Verification items for this drawing (mm, ordinates from the low corner). A direction names the side the tool comes from. Round coordinates to 2 decimals unless told otherwise and drop trailing zeros. Loops run counter-clockwise (first coordinate to the right, second up) from the corner with the lowest first, then second, coordinate; pieces in that order, holes last. Notation, with made-up numbers: (-20.75, 56.25) - (8.25, 56.25) arc R17 cw to (8.25, 80.25) - close; hole circle Ø7 at (14.5, 34.5). An arc over 180 degrees is marked (long way). Put each result on its own line as item: value.
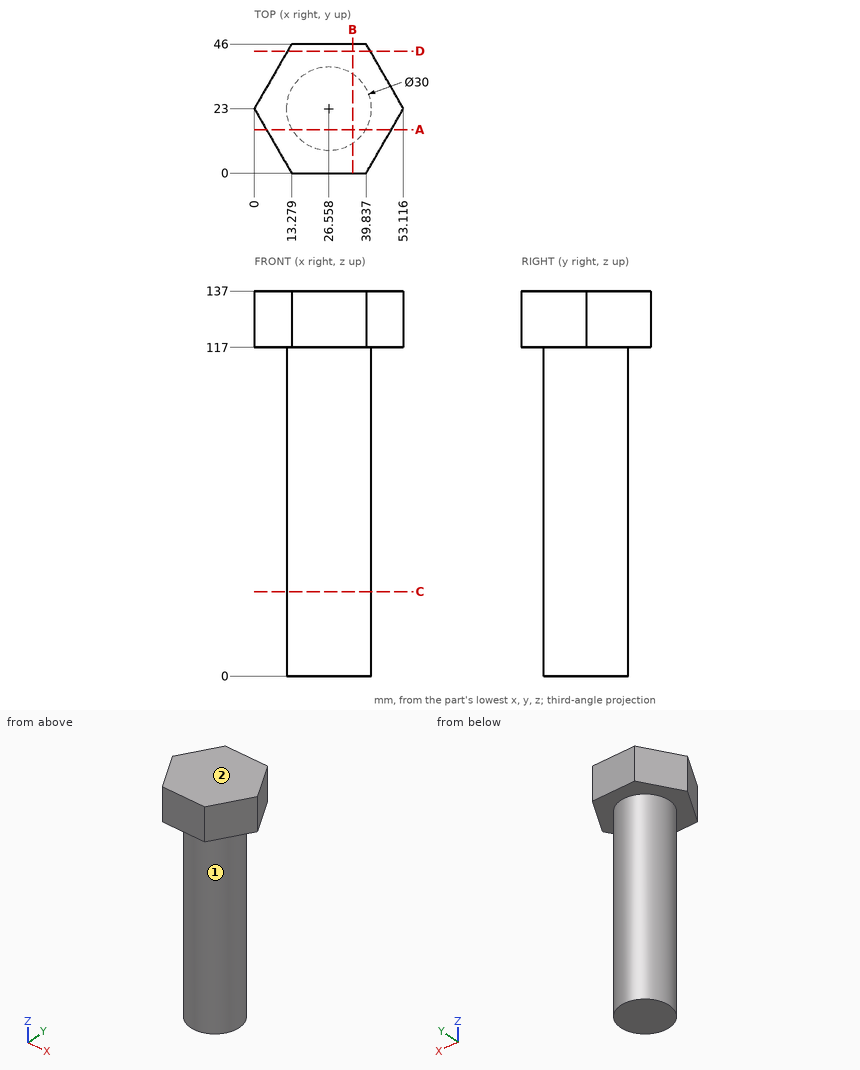
Item 1: Section check B-B on x = 35. Enter the section's corners in (y, z), then the cut area to 3 significant figures.
Filled sheet:
outline: (0, 117) - (10.6, 117) - (10.6, 0) - (35.4, 0) - (35.4, 117) - (46, 117) - (46, 137) - (0, 137) - close
area: 3,820 mm²
Item 2: Tool access check on the marked faces 1 and 2. Record the directions out of +Z, -Z, +X, -X, +Y, -Y that give a thin tool (end or side, any length) a straight path to the whole face; none if there is none.
Filled sheet:
face 1: -Z
face 2: +Z, +X, -X, +Y, -Y
Item 3: Thickness scan on line 1 (Z direction, x = 7, y = 30.5); line 2 (X direction, y = 32.5, z = 26.5); line 3 (Y direction, x = 19, z = 31). Record the ranges inside material, lowest first. Write a range as from..to.
Filled sheet:
line 1: 117..137
line 2: 14.95..38.17
line 3: 10.04..35.96
Item 4: Section check C-C on z = 30. Enter the section's corners in (x, y).
Filled sheet:
outline: circle Ø30 at (26.56, 23)
Item 5: Section check A-A on y = 15.5. Enter the section's corners in (x, z).
Filled sheet:
outline: (4.33, 117) - (13.57, 117) - (13.57, 0) - (39.55, 0) - (39.55, 117) - (48.79, 117) - (48.79, 137) - (4.33, 137) - close
Item 6: Go/stop test with flat-tipped pins: pin 1 (10 mm diameter, centred on x = 16.5, z = 39.5, fed in from +Y); pin 2 (1.5 mm diameter, centred on x = 20.5, y = 5, fed in from -Z); pin 3 (4 mm diameter, centred on x = 24, z = 78, fed in from -Y). Record where each tip stops, or that it passes through.
Filled sheet:
pin 1: y = 37.12
pin 2: z = 117
pin 3: y = 8.01
Item 7: Section check D-D on y = 43.5. Enter the section's corners in (x, z).
Filled sheet:
outline: (11.84, 117) - (41.28, 117) - (41.28, 137) - (11.84, 137) - close
